Here's how the part is built. I have some questions about the finished solid (model axes, mm). A direction names the side the tool comes from. Coordinates: 2 decimals unless noted, no trailing zeros. Order: outer loops, then holes, each group sorted by start corner. A loop starts at its lowest first (then second) coordinate and runs counter-clockwise, first axis right, second up. Notation, with made-up numbers: (-8.5, 34.5) -> (39.5, 34.5) arc R20 cw to (39.5, 70.5) -> close; hole circle Ø5 at (37, 29). An arc over 180 degrees is marked (long way). One line per item, written item: value. Start each with the question number.
```python
from build123d import *

# Parameters (mm, degrees)
F2_DEPTH = 6.4


with BuildPart() as f2:
    # F1 (on Top) → F2 (new body)
    with BuildSketch(Plane.XY):
        with BuildLine():
            Line((-46.5, 4.3), (-46.5, -78.05))
            ThreePointArc((-46.5, -78.05), (-44.7426406871, -82.2926406871), (-40.5, -84.05))
            Line((-40.5, -84.05), (-34.1, -84.05))
            add(Edge.make_bspline(
                [(-34.1, -84.05), (46.5, -84.05), (46.5, -4.3)],
                knots=[4.7123889804, 4.7123889804, 4.7123889804, 6.2831853072, 6.2831853072, 6.2831853072], degree=2, weights=[1, 0.7071067812, 1]))
            ThreePointArc((46.5, -4.3), (31.6210244843, 31.6210244843), (-4.3, 46.5))
            ThreePointArc((-4.3, 46.5), (-34.1399061661, 34.1399061661), (-46.5, 4.3))
        make_face()
        with BuildLine():
            Line((-34.1, -78.05), (-40.5, -78.05))
            Line((-40.5, -78.05), (-40.5, -20.05))
            Line((-40.5, -20.05), (-34.1, -20.05))
            Line((-34.1, -20.05), (-34.1, -25.9702287672))
            ThreePointArc((-34.1, -25.9702287672), (-28.5967900968, -22.2326106882), (-30.0422633054, -15.7390973598))
            ThreePointArc((-30.0422633054, -15.7390973598), (-36.4430153205, -6.6146899597), (-38.7, 4.3))
            ThreePointArc((-38.7, 4.3), (-28.6244732728, 28.6244732728), (-4.3, 38.7))
            ThreePointArc((-4.3, 38.7), (26.105591591, 26.105591591), (38.7, -4.3))
            ThreePointArc((38.7, -4.3), (22.9569894888, -42.3069894888), (-15.05, -58.05))
            Line((-15.05, -58.05), (-28.1, -58.05))
            ThreePointArc((-28.1, -58.05), (-32.3426406871, -59.8073593129), (-34.1, -64.05))
            Line((-34.1, -64.05), (-34.1, -78.05))
        make_face(mode=Mode.SUBTRACT)
    extrude(amount=F2_DEPTH)


solid = f2.part
```
Q1. For faces 5 (the face through (-32, -18, 6.4)), 6 (the face through (-32.296, -59.761, 3.155)), which set-ups out of +Z, -Z, +X, -X, +Y, -Y let a thin tool reach every point of the face, with its end or its side?
Q2. For P1, Ø1.9, axis at x = -19, z = 4.5, coming from the +Y side, with a flat end and sliding along its axis, tell me the tip position at first contact or that it passes through.
Q3. Imagine slicing it at B-B (y = 17.5). Write out the boundary of the cut face in (x, z).
Q4. If we mould it in two halves opening along Y, with no side actions, what happens to faces 1 (the face through (-28.634, -22.324, 3.155)), 2 (the face through (-44.789, -82.246, 3.155)), 3 (the face through (32.014, 31.224, 3.155)), 4 (the face through (-28.89, 28.356, 3.155))? For each: +Y half, -Y half, draft (parallel to the pull), parting line (faces both ways), or undercut.
Q5. I need wall thicknesses on line 1 (Y direction, x = 10, z = 5.5); line 2 (X direction, y = -38, z = 3.25); line 3 (X direction, y = -51.5, z = 1.5). Which ranges of each line are inside material? Lowest first, please.
Q6. Imagine slicing it at A-A (y = 2). Write out the boundary of the cut face in (x, z), plus the area to 3 significant figures.
Completed:
1. face 5: +Z, +X, -X, +Y, -Y
1. face 6: +Z, -Z
2. P1: stops at y = 44.2
3. outline: (-44.38, 0) -> (-36.07, 0) -> (-36.07, 6.4) -> (-44.38, 6.4) -> close; (32.76, 0) -> (41.58, 0) -> (41.58, 6.4) -> (32.76, 6.4) -> close
4. face 1: undercut
4. face 2: -Y half
4. face 3: +Y half
4. face 4: undercut
5. line 1: y = -71.05 to -51.86, 36.25 to 44.45
5. line 2: x = -46.5 to -40.5, 26.82 to 38.95
5. line 3: x = -46.5 to -40.5, 10.66 to 30.87
6. outline: (-46.5, 0) -> (-38.6, 0) -> (-38.6, 6.4) -> (-46.5, 6.4) -> close; (38.24, 0) -> (46.11, 0) -> (46.11, 6.4) -> (38.24, 6.4) -> close
6. area: 101 mm2
